For this review, take the finished solid that the model builds, in its own axes (mm). A direction names the side the tool comes from. Round coordinates to 2 decimals unless told otherwise and drop trailing zeros. Loops run counter-clockwise (first coordinate to the right, second up) from the corner with the lowest first, then second, coordinate; pieces in that order, holes last.
1) Insertion check: pin 1 (12 mm diameter, centred on x = 34, y = 45.5, fed in from +Z); pin 2 (3.5 mm diameter, centred on y = 46, z = 3, fed in from +X); pin 3 (2 mm diameter, centred on x = 23, z = 5.5, fed in from +Y); pin 4 (2 mm diameter, centred on x = 55, z = 2, fed in from +Y). Each pin has a flat end and moves straight along its axis. Give the tip position at first contact, or say it passes through.
2) Take a section at B-B (y = 28.5). State the section outline as (x, z) points.
3) Take a section at A-A (x = 52.5). State the section outline as (y, z) points, then the cut area to 3 significant figures.
4) Wall thickness on L1, parallel to Y at x = 45.5, z = 0.5; L2, parallel to X at y = 3, z = 2; L3, parallel to X at y = 14.5, z = 5.25: over which ranges is each line inside the solid? List them lowest first.
5) Mouldability with a two-part tool opening along X and no side actions: class faces 4 (the flat face through (41.542, 49.332, 3.413)), 5 (the flat face through (42.37, 52.66, 3.32)), 6 (the flat face through (53, 40, 3)) as pulls with the +X half, pulls with the -X half, needs draft (parallel to the pull), parting line crosses it, or undercut.
6) Tool access review of faces 1 (the flat face through (53, 20, 3)), 2 (the flat face through (32.32, 43.73, 3.32)), 3 (the flat face through (45.694, 42.237, 3.413)): name each direction out of +Z, -Z, +X, -X, +Y, -Y from which nothing blocks a thin tool from reaching the whole face with its end or side.
Autodesk Inventor part; units mm, degrees
ref_plane "YZ Plane" through (0, 0, 0) normal (1, 0, 0) x (0, 1, 0)
ref_plane "XZ Plane" through (0, 0, 0) normal (0, 1, 0) x (-1, 0, 0)
ref_plane "XY Plane" through (0, 0, 0) normal (0, 0, 1) x (1, 0, 0)
sketch "Sketch1" plane through (0, 0, 0) normal (0, 0, 1) x (1, 0, 0)
  line L0 (0, 0) -> (50, 0)
  line L1 (50, 0) -> (50, 40)
  line L2 (50, 40) -> (56.731, 40)
  line L3 (56.731, 40) -> (56.731, 20)
  line L4 (56.731, 20) -> (50, 20)
  line L5 (50, 20) -> (50, 40)
  line L6 (10, 3.269) -> (30, 3.269)
  line L7 (30, 3.269) -> (30, 10)
  line L8 (30, 10) -> (10, 10)
  line L9 (10, 10) -> (10, 3.269)
  line L10 (0, 10) -> (10, 10)
  line L11 (30, 10) -> (50, 10)
  line L12 (0, 10) -> (0, 0)
  line L13 (0, 10) -> (0, 15)
  line L14 (0, 15) -> (45, 55)
  line L15 (50, 40) -> (50, 55)
  line L16 (50, 55) -> (45, 55)
  point P0 (20, 3.269)
  point P1 (20, 0)
  dimension "d2" = 20
  dimension "d3" = 20
  dimension "d5" = 6.731
  dimension "d6" = 10
  dimension "d9" = 10
  dimension "d11" = 20
  dimension "d12" = 20
  dimension "d14" = 5
  dimension "d16" = 15
  dimension "d17" = 5
extrude "Extrusion1" add sketch "Sketch1" along normal blind 6.731
sketch "Sketch2" plane through (0, 0, 6.731) normal (0, 0, 1) x (1, 0, 0)
  line L0 (45, 55) -> (0, 15)
  line L1 (4.4845, 18.9862) -> (6.5938, 16.6132)
  line L2 (6.5938, 16.6132) -> (29.0161, 36.5441)
  line L3 (29.0161, 36.5441) -> (26.9067, 38.9171)
  dimension "d18" = 3.175
  dimension "d19" = 30
  dimension "d20" = 6
extrude "Extrusion2" cut sketch "Sketch2" against normal up to next
fillet "Fillet1" radius 1.5875 4 edges at (45, 55, 3.3655) (0, 0, 3.3655) (6.5938, 16.6132, 3.3655) (29.0161, 36.5441, 3.3655)
sketch "Sketch3" plane through (0, 0, 6.731) normal (0, 0, 1) x (1, 0, 0)
  line L0 (45, 55) -> (0, 15)
  line L1 (3.2333, 17.874) -> (5.7738, 15.0159)
  line L2 (5.7738, 15.0159) -> (6.8292, 15.954)
  line L3 (6.8292, 15.954) -> (8.9392, 13.5803)
  line L4 (8.9392, 13.5803) -> (7.8838, 12.6422)
  line L5 (7.8838, 12.6422) -> (9.8769, 10.3999)
  line L6 (9.8769, 10.3999) -> (7.5032, 8.2899)
  line L7 (7.5032, 8.2899) -> (5.5101, 10.5322)
  line L8 (5.5101, 10.5322) -> (4.4547, 9.5941)
  line L9 (4.4547, 9.5941) -> (2.3447, 11.9678)
  line L10 (2.3447, 11.9678) -> (3.4, 12.9059)
  line L11 (3.4, 12.9059) -> (0.8595, 15.764)
  line L12 (37.8802, 48.6713) -> (40.4207, 45.8132)
  line L13 (40.4207, 45.8132) -> (39.3654, 44.8751)
  line L14 (39.3654, 44.8751) -> (41.4754, 42.5013)
  line L15 (41.4754, 42.5013) -> (42.5307, 43.4394)
  line L16 (42.5307, 43.4394) -> (44.5238, 41.1972)
  line L17 (44.5238, 41.1972) -> (46.8976, 43.3072)
  line L18 (46.8976, 43.3072) -> (44.9045, 45.5494)
  line L19 (44.9045, 45.5494) -> (45.9598, 46.4875)
  line L20 (45.9598, 46.4875) -> (43.8498, 48.8613)
  line L21 (43.8498, 48.8613) -> (42.7945, 47.9232)
  line L22 (42.7945, 47.9232) -> (40.254, 50.7813)
  dimension "d24" = 3.176
  dimension "d25" = 10
  dimension "d26" = 3
  dimension "d27" = 6
  dimension "d28" = 1.15
  dimension "d29" = 6.35
extrude "Extrusion3" cut sketch "Sketch3" against normal up to next
equation "\"d5\" = THICKB"
equation "\"d7\" = THICKB"
equation "\"THICKA\" = 3.175"
equation "\"THICKB\" = 6.731"
equation "\"THICKC\" = 12.7"
equation "\"THICKPLY\" = 5"
equation "\"MAGDIA\" = 9.5"
equation "\"BALLDIA\" = 12"
properties part number "Mount_LCD_End_SD"
Response:
1. pin 1: stops at z = 6.73
1. pin 2: stops at x = 50
1. pin 3: stops at y = 32.09
1. pin 4: stops at y = 40
2. outline: (19.97, 0) - (56.73, 0) - (56.73, 6.73) - (19.97, 6.73) - close
3. outline: (20, 0) - (40, 0) - (40, 6.73) - (20, 6.73) - close
3. area: 135 mm2
4. L1: y = 0 to 42.06, 44.88 to 46.08, 47 to 55
4. L2: x = 0 to 50
4. L3: x = 0 to 1.98, 8.12 to 50
5. face 4: undercut
5. face 5: pulls with the -X half
5. face 6: needs draft
6. face 1: +Z, -Z, +X, -Y
6. face 2: +Z, -Z, -X, +Y
6. face 3: +Z, -Z
